```python
from build123d import *

# Parameters (mm, degrees)
SKETCH1_R  = 1
BODY_DEPTH = 1
FILLET1_R  = 0.5
FILLET2_R  = 1


with BuildPart() as part:
    # Sketch1 → Body (new body)
    with BuildSketch(Plane.XY):
        with BuildLine():
            Line((-1.25, -9.83515139), (-1.25, -13.911129106))
            ThreePointArc((-1.25, -13.911129106), (-4.193699318, -13.291524711), (-6.922858868, -12.026232874))
            Line((-6.922858868, -12.026232874), (-7.577141132, -8.315613763))
            ThreePointArc((-7.577141132, -8.315613763), (0, 11.25), (7.577141132, -8.315613763))
            Line((7.577141132, -8.315613763), (6.922858868, -12.026232874))
            ThreePointArc((6.922858868, -12.026232874), (4.193699318, -13.291524711), (1.25, -13.911129106))
            Line((1.25, -13.911129106), (1.25, -9.83515139))
            ThreePointArc((1.25, -9.83515139), (0, 8.58), (-1.25, -9.83515139))
        make_face()
        with Locations((4.25, -11.032311518)):
            Circle(SKETCH1_R, mode=Mode.SUBTRACT)
        with Locations((-4.25, -11.032311518)):
            Circle(SKETCH1_R, mode=Mode.SUBTRACT)
    extrude(amount=-BODY_DEPTH)

    # Fillet1
    fillet1_edges = [part.edges().sort_by_distance(p)[0] for p in [
        (-6.922858868, -12.026232874, -0.5),
        (6.922858868, -12.026232874, -0.5),
    ]]
    fillet(fillet1_edges, radius=FILLET1_R)

    # Fillet2
    fillet2_edges = [part.edges().sort_by_distance(p)[0] for p in [
        (-7.577141132, -8.315613763, -0.5),
        (7.577141132, -8.315613763, -0.5),
    ]]
    fillet(fillet2_edges, radius=FILLET2_R)


solid = part.part
```
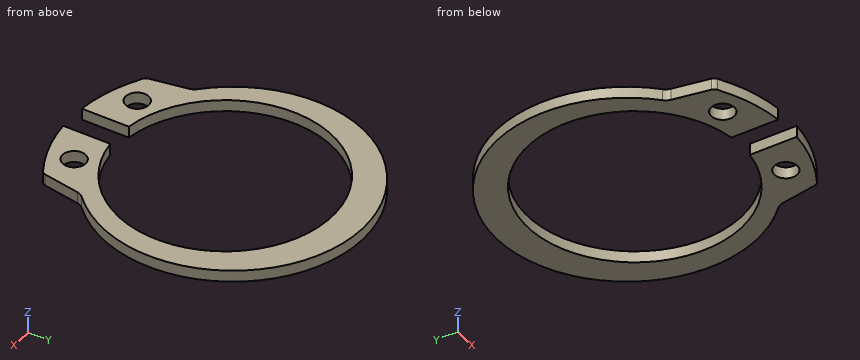
Geometry check sheet. Reference: the model listing, model coordinates, mm. Round coordinates to 2 decimals unless told otherwise and drop trailing zeros. Order: outer loops, then holes, each group sorted by start corner. A loop starts at its lowest first (then second) coordinate and runs counter-clockwise, first axis right, second up. Notation, with made-up numbers: (-26.5, 30.5) -> (4.5, 30.5) arc R21 cw to (4.5, 65.5) -> close; hole circle Ø4 at (6, 41.5). An arc over 180 degrees is marked (long way). Return JSON: item names as keys, results as strings. Group by question number.
Q1. Gauge pin test, flat end, axial feed: pin 1 (1.8 mm diameter, centred on x = 4.25, y = -11.03, fed in from -Z). Record the tip position at first contact, or that the pin passes through.
Q2. Section check B-B, the plane y = 0. Record the boundary of the cut face in (x, z).
Q3. Section check D-D, the plane y = -5.25. Record the boundary of the cut face in (x, z).
Q4. Material ranges on probe 1 along X at (y, z) = (-11.75, -0.35); probe 2 along Y at (x, z) = (4.25, -0.55); probe 3 along Y at (x, z) = (0, -0.35), recorded low to high. Write a range as from..to.
Q5. Section check C-C, the plane z = -0.55. Record the boundary of the cut face in (x, y).
Q6. Section check A-A, the plane x = 4.25. Record the boundary of the cut face in (y, z), plus the area to 3 significant figures.
Numbers:
{
 "1": {"pin 1": "through"},
 "2": {"outline": "(-11.25, -1) -> (-9.23, -1) -> (-9.23, 0) -> (-11.25, 0) -> close; (9.23, -1) -> (11.25, -1) -> (11.25, 0) -> (9.23, 0) -> close"},
 "3": {"outline": "(-9.95, -1) -> (-8.04, -1) -> (-8.04, 0) -> (-9.95, 0) -> close; (8.04, -1) -> (9.95, -1) -> (9.95, 0) -> (8.04, 0) -> close"},
 "4": {"probe 1": "-6.97..-4.95, -3.55..-1.25, 1.25..3.55, 4.95..6.97", "probe 2": "-13.27..-12.03, -10.03..-8.89, 7.55..10.42", "probe 3": "8.58..11.25"},
 "5": {"outline": "(-7.81, -8.1) arc R1 cw to (-7.52, -8.64) -> (-6.96, -11.8) arc R0.5 ccw to (-6.72, -12.15) arc R13.3 ccw to (-1.25, -13.91) -> (-1.25, -9.84) arc R9.25 cw (long way) to (1.25, -9.84) -> (1.25, -13.91) arc R13.3 ccw to (6.72, -12.15) arc R0.5 ccw to (6.96, -11.8) -> (7.52, -8.64) arc R1 cw to (7.81, -8.1) arc R11.25 ccw (long way) to start; hole circle Ø2 at (-4.25, -11.03); hole circle Ø2 at (4.25, -11.03)"},
 "6": {"outline": "(-13.27, -1) -> (-12.03, -1) -> (-12.03, 0) -> (-13.27, 0) -> close; (-10.03, -1) -> (-8.89, -1) -> (-8.89, 0) -> (-10.03, 0) -> close; (7.55, -1) -> (10.42, -1) -> (10.42, 0) -> (7.55, 0) -> close", "area": "5.26 mm^2"}
}
